from build123d import *

# Parameters (mm, degrees)
SKETCH2_R           = 12.7
SKETCH2_R_2         = 11.43
BOSS_EXTRUDE1_DEPTH = 53.34
SKETCH3_R           = 12.7
SKETCH3_R_2         = 11.43
BOSS_EXTRUDE2_DEPTH = 12.7
BOSS_EXTRUDE3_START = 12.7
SKETCH4_R           = 12.7
SKETCH4_R_2         = 11.43
BOSS_EXTRUDE3_DEPTH = 12.7
SKETCH5_R           = 11.43
CUT_EXTRUDE1_DEPTH  = 25.4
SKETCH6_R           = 11.43
CUT_EXTRUDE2_DEPTH  = 61.428516577


with BuildPart() as part:
    # Sketch2 → Boss-Extrude1 (new body)
    with BuildSketch(Plane.XY):
        Circle(SKETCH2_R)
        Circle(SKETCH2_R_2, mode=Mode.SUBTRACT)
    extrude(amount=BOSS_EXTRUDE1_DEPTH)

    # Sketch3 → Boss-Extrude2 (add)
    with BuildSketch(Plane(origin=(12.7, 0, 0), x_dir=(0, 0, -1), z_dir=(1, 0, 0))):
        with Locations((-26.67, 0)):
            Circle(SKETCH3_R)
        with Locations((-26.67, 0)):
            Circle(SKETCH3_R_2, mode=Mode.SUBTRACT)
    extrude(amount=-BOSS_EXTRUDE2_DEPTH)

    # Sketch4 → Boss-Extrude3 (add)
    with BuildSketch(Plane(origin=(12.7, 0, 0), x_dir=(0, 0, -1), z_dir=(1, 0, 0)).offset(BOSS_EXTRUDE3_START)):
        with Locations((-26.67, 0)):
            Circle(SKETCH4_R)
        with Locations((-26.67, 0)):
            Circle(SKETCH4_R_2, mode=Mode.SUBTRACT)
    extrude(amount=-BOSS_EXTRUDE3_DEPTH)

    # Sketch5 → Cut-Extrude1 (cut)
    with BuildSketch(Plane(origin=(25.4, 0, 0), x_dir=(0, 0, -1), z_dir=(1, 0, 0))):
        with Locations((-26.67, 0)):
            Circle(SKETCH5_R)
    extrude(amount=-CUT_EXTRUDE1_DEPTH, mode=Mode.SUBTRACT)

    # Sketch6 → Cut-Extrude2 (cut, through all)
    with BuildSketch(Plane(origin=(0, 0, 0), x_dir=(-1, 0, 0), z_dir=(0, 0, -1))):
        with Locations(Location((0, 0, 0), (0, 0, 180))):
            Circle(SKETCH6_R)
    extrude(amount=-CUT_EXTRUDE2_DEPTH, mode=Mode.SUBTRACT)


solid = part.part
Here's how the part is built. I have some questions about the finished solid (model axes, mm). Round coordinates to 2 decimals unless told otherwise and drop trailing zeros. Write each loop counter-clockwise with the first axis right and the second up, starting at its lowest first coordinate (ties: lowest second). Pieces come first, ordered by that corner, then holes.
1. Will these pins go through, and if not, where does the flat tip stop? pin 1 Ø6 at (y, z) = (2.5, 35) entering from +X; pin 2 Ø10 at (x, z) = (10, 37) entering from -Y; pin 3 Ø1 at (y, z) = (9, 7) entering from -X; pin 4 Ø3 at (x, z) = (15, 8.5) entering from +Y.
2. Suppose I cut it at C-C (x = -6). List the corners of the cut face in (y, z) for me, and give its area (3 significant figures).
3. If we mould it in two halves opening along Y, with no side actions, what happens to faces 1 (the flat face through (25.4, 7, 36)), 2 (the cylindrical face through (-11.42, 0.5, 26.3)), 3 (the cylindrical face through (15.7, 10.709, 19.843))? For each: released by +Y, released by -Y, zero draft, split by the parting line, or undercut.
4. Suppose I cut it at A-A (y = 0). List the corners of the cut face in (x, z) for me.
5. Suppose I cut it at D-D (y = -8.5). List the corners of the cut face in (x, z) for me.
6. Suppose I cut it at B-B (z = 26.67). List the corners of the cut face in (x, y) for me, and give its area (3 significant figures).
7. I need wall thicknesses on L1, parallel to Y at x = 5, z = 26.67; L2, parallel to Y at x = 3, z = 38; L3, parallel to X at y = -9.25, z = 47.5. Which ranges of each line are inside material? Lowest first, please.
Answer sheet:
1. pin 1: stops at x = 25.4
1. pin 2: stops at y = -11.67
1. pin 3: stops at x = -9.44
1. pin 4: passes through
2. outline: (-11.19, 0) - (-9.73, 0) - (-9.73, 53.34) - (-11.19, 53.34) - close; (9.73, 0) - (11.19, 0) - (11.19, 53.34) - (9.73, 53.34) - close
2. area: 156 mm2
3. face 1: zero draft
3. face 2: undercut
3. face 3: split by the parting line
4. outline: (-12.7, 0) - (-11.43, 0) - (-11.43, 53.34) - (-12.7, 53.34) - close; (11.43, 0) - (12.7, 0) - (12.7, 13.97) - (25.4, 13.97) - (25.4, 15.24) - (11.43, 15.24) - close; (11.43, 38.1) - (25.4, 38.1) - (25.4, 39.37) - (12.7, 39.37) - (12.7, 53.34) - (11.43, 53.34) - close
5. outline: (-9.44, 0) - (-7.64, 0) - (-7.64, 53.34) - (-9.44, 53.34) - close; (7.64, 0) - (9.44, 0) - (9.44, 17.23) - (25.4, 17.23) - (25.4, 19.03) - (7.64, 19.03) - close; (7.64, 34.31) - (25.4, 34.31) - (25.4, 36.11) - (9.44, 36.11) - (9.44, 53.34) - (7.64, 53.34) - close
6. outline: (0, -12.7) - (25.4, -12.7) - (25.4, -11.43) - (0, -11.43) arc R11.43 cw to (0, 11.43) - (25.4, 11.43) - (25.4, 12.7) - (0, 12.7) arc R12.7 ccw to start
6. area: 113 mm2
7. L1: y = -12.7 to -11.43, 11.43 to 12.7
7. L2: y = -12.34 to -11.03, 11.03 to 12.34
7. L3: x = -8.7 to -6.71, 6.71 to 8.7
